from build123d import *

# Parameters (mm, degrees)
F0_W     = 88.9
F0_H     = 69.85
F0_W_2   = 85.725
F0_H_2   = 66.675
F1_DEPTH = 3.175
F0_W_3   = 74.6125
F0_H_3   = 55.5625
F2_DEPTH = 6.35
F0_W_4   = 50.8
F0_H_4   = 50.8
F3_DEPTH = 6.35
F4_DEPTH = 1.5875


with BuildPart() as f1:
    # F0 (on Top) → F1 (new body)
    with BuildSketch(Plane.XY):
        Rectangle(F0_W, F0_H)
        Rectangle(F0_W_2, F0_H_2, mode=Mode.SUBTRACT)
    extrude(amount=F1_DEPTH)

    # F0 (on Top) → F2 (join)
    with BuildSketch(Plane.XY):
        Rectangle(F0_W_2, F0_H_2)
        Rectangle(F0_W_3, F0_H_3, mode=Mode.SUBTRACT)
    extrude(amount=F2_DEPTH)

    # F0 (on Top) → F3 (join)
    with BuildSketch(Plane.XY):
        Rectangle(F0_W_3, F0_H_3)
        Rectangle(F0_W_4, F0_H_4, mode=Mode.SUBTRACT)
    extrude(amount=F3_DEPTH)

    # F0 (on Top) → F4 (cut, symmetric)
    with BuildSketch(Plane.XY):
        Rectangle(F0_W_3, F0_H_3)
        Rectangle(F0_W_4, F0_H_4, mode=Mode.SUBTRACT)
    extrude(amount=F4_DEPTH, both=True, mode=Mode.SUBTRACT)


solid = f1.part
The model under review builds one solid part; all positions refer to its coordinate system, in mm. A direction names the side the tool comes from. Give positions to 0.01 mm unless a question says otherwise; leave off trailing zeros. Order: outer loops, then holes, each group sorted by start corner. A loop starts at its lowest first (then second) coordinate and runs counter-clockwise, first axis right, second up. Notation, with made-up numbers: M 33.5,27.25 L 54.5,27.25 A6 cw 54.5,34.25 Z; hole C 27,-21 d4. An arc over 180 degrees is marked long. Answer in a Markdown table with one row per item. Add a question column.
1. To check wall thickness, follow line 1 along Y through (x, z) = (20, 6); line 2 along X through (y, z) = (-11, 1.25); line 3 along X through (y, z) = (24, 2). State the ranges of each line that lie inside material, in increasing order.
2. Machinability: for faces 1 (the flat face through (-42.862, 0, 5)), 2 (the flat face through (-25.4, 0, 4)), 3 (the flat face through (-1, -33.338, 5)), 4 (the flat face through (42.862, 0, 5)), which of the approach directions +Z, -Z, +X, -X, +Y, -Y give a long, thin tool a straight path to every point of the face, cutting with its end or side? Answer none if there is none.
3. For pin 1 Ø1.5 at (y, z) = (-21, 4) entering from -X; pin 2 Ø2.5 at (y, z) = (-6.5, 5) entering from +X; pin 3 Ø2 at (x, y) = (5, 26.5) entering from -Z, all flat-tipped, find the tip position at first contact; note any pin that passes through.
4. Add section B-B on z = 4.5. State the section outline as (x, y) points, plus the area to 3 significant figures.
5. Mouldability with a two-part tool opening along X and no side actions: class faces 5 (the flat face through (0, 25.4, 4)), 6 (the flat face through (-44.45, 0, 2)), 7 (the flat face through (44.45, 0, 2)) as released by +X, released by -X, zero draft, split by the parting line, or undercut.
The answers:
| question | item | result |
|---|---|---|
| 1 | line 1 | -33.34 to -25.4, 25.4 to 33.34 |
| 1 | line 2 | -44.45 to -37.31, 37.31 to 44.45 |
| 1 | line 3 | -44.45 to -25.4, 25.4 to 44.45 |
| 2 | face 1 | +Z, -X, +Y, -Y |
| 2 | face 2 | +Z, -Z |
| 2 | face 3 | +Z, +X, -X, -Y |
| 2 | face 4 | +Z, +X, +Y, -Y |
| 3 | pin 1 | x = -42.86 |
| 3 | pin 2 | x = 42.86 |
| 3 | pin 3 | z = 1.59 |
| 4 | outline | M -42.86,-33.34 L 42.86,-33.34 L 42.86,33.34 L -42.86,33.34 Z; hole M -25.4,-25.4 L 25.4,-25.4 L 25.4,25.4 L -25.4,25.4 Z |
| 4 | area | 3,140 mm2 |
| 5 | face 5 | undercut |
| 5 | face 6 | released by -X |
| 5 | face 7 | released by +X |
